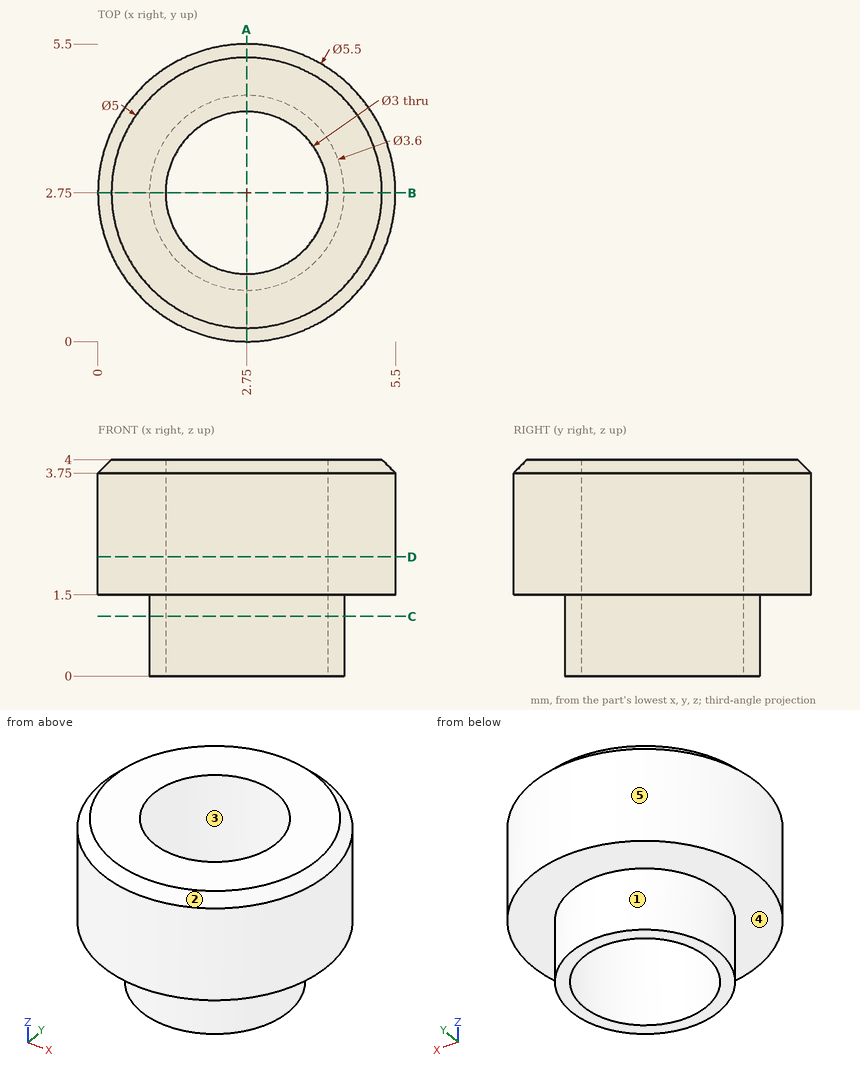
Geometry check sheet. Reference: drawing and pictorial views, mm from the part's lowest x, y, z. A direction names the side the tool comes from. Round coordinates to 2 decimals unless told otherwise and drop trailing zeros. Order: outer loops, then holes, each group sorted by start corner. A loop starts at its lowest first (then second) coordinate and runs counter-clockwise, first axis right, second up. Notation, with made-up numbers: M 43,6 L 73,6 A36 cw 73,40 Z; hole C -30,-14.5 d6. An arc over 180 degrees is marked long. Answer as CSV lines item,"result".
1) Tool access check on the marked faces 1 and 2. Record the directions out of +Z, -Z, +X, -X, +Y, -Y that give a thin tool (end or side, any length) a straight path to the whole face; none if there is none.
Entries:
face 1,"-Z"
face 2,"+Z"
2) Mould release check, pull along Y, two halves, no side actions. Record for the marked faces 3, 4 and 5: +Y half, -Y half, draft (parallel to the pull), parting line (faces both ways), or undercut.
Entries:
face 3,"undercut"
face 4,"draft"
face 5,"parting line"
3) Thickness scan on probe 1 along X at (y, z) = (2.75, 1); probe 2 along X at (y, z) = (2.75, 2.9). Record the ranges inside material, lowest first. Write a range as [from, to].
Entries:
probe 1,"[0.95, 1.25], [4.25, 4.55]"
probe 2,"[0, 1.25], [4.25, 5.5]"
4) Sectioned sample at A-A on x = 2.75. Record the cut outline in (y, z), and give its area (3 significant figures).
Entries:
outline,"M 0,1.5 L 0.95,1.5 L 0.95,0 L 1.25,0 L 1.25,4 L 0.25,4 L 0,3.75 Z; M 4.25,0 L 4.55,0 L 4.55,1.5 L 5.5,1.5 L 5.5,3.75 L 5.25,4 L 4.25,4 Z"
area,"7.09 mm2"
5) Sectioned sample at D-D on z = 2.2. Record the cut outline in (x, y), and give its area (3 significant figures).
Entries:
outline,"C 2.75,2.75 d5.5; hole C 2.75,2.75 d3"
area,"16.7 mm2"
6) Sectioned sample at C-C on z = 1.1. Record the cut outline in (x, y), and give its area (3 significant figures).
Entries:
outline,"C 2.75,2.75 d3.6; hole C 2.75,2.75 d3"
area,"3.11 mm2"
